Autodesk Inventor part; units mm, degrees
ref_plane "Work Plane1" through (104.775, 0, 0) normal (0, 0, -1) x (1, 0, 0)
ref_plane "YZ Plane" through (0, 0, 0) normal (1, 0, 0) x (0, 1, 0)
ref_plane "XZ Plane" through (0, 0, 0) normal (0, 1, 0) x (-1, 0, 0)
sketch "Sketch1" plane through (0, 0, 0) normal (0, 0, 1) x (1, 0, 0)
  line L0 (15.875, 0) -> (15.875, 2.413)
  line L1 (15.875, 2.413) -> (5.8717, 2.413)
  line L2 (5.8717, 2.413) -> (3.2258, 2.413)
  line L3 (0, 4.5593) -> (0, 1.8331)
  line L4 (0, 1.8331) -> (2.2098, 1.8331)
  line L5 (2.2098, 1.8331) -> (3.2681, 0)
  line L6 (3.2681, 0) -> (15.875, 0)
  line L7 (0, 4.5593) -> (0.7568, 4.5593)
  line L8 (0.7568, 4.5593) -> (3.2258, 2.413)
  line L9 (3.2258, 2.413) -> (3.2258, 2.413)
  line L10 (5.8717, 2.413) -> (3.2258, 2.413) construction
  line L11 (3.2258, 2.413) -> (3.2258, 2.413)
  line L12 (-3.175, 0) -> (19.05, 0)
  line L13 (0, -0.9119) -> (0, 5.4712)
  dimension "d0" = 15.875
  dimension "d1" = 10.0033
  dimension "d2" = 2.2098
  dimension "d3" = 4.826
  dimension "d6" = 3.2258
  dimension "d7" = 41
  dimension "d8" = 3.6662
  dimension "d9" = 60
  dimension "d10" = 9.1186
  dimension "d11" = 4.826
  dimension "d12" = 2.6459
revolve "Body" add sketch "Sketch1" angle 360 about axis through (3.2681, 0, 0) along (1, 0, 0) contours L6 L5 L4 L3 L7 L8 L2 L1 L0
sketch "Sketch2" plane through (0, 0, 0) normal (-1, 0, 0) x (0, 0, 1)
  circle A0 centre (0, 0) radius 1.8331
  line L0 (0, -6.383) -> (0, 6.383)
  line L1 (-6.383, 0) -> (6.383, 0)
  line L2 (1.8331, 0) -> (0.9165, -1.5875)
  line L3 (0.9165, -1.5875) -> (-0.9165, -1.5875)
  line L4 (-0.9165, -1.5875) -> (-1.8331, 0)
  line L5 (-1.8331, 0) -> (-0.9165, 1.5875)
  line L6 (-0.9165, 1.5875) -> (0.9165, 1.5875)
  line L7 (0.9165, 1.5875) -> (1.8331, 0)
  point P0 (0, 1.8331)
extrude "Slot" add sketch "Sketch2" against normal up to next contours L7 A0 | A0 L2 | L6 L0 A0 | A0 L0 L3 | L0 L6 A0 | A0 L3 L0 | L4 A0 | A0 L5
thread "Thread"
chamfer "Chamfer1" distance 0.6299 distance2 1.2598 1 edges at (15.875, -2.413, 0) measured on face at (15.875, -0.0132, -0.958)
ref_plane "Work Plane1" through (104.775, 0, 0) normal (0, 0, -1) x (1, 0, 0)
equation "\"d15\" = GEL"
equation "\"d17\" = -0.5 * SPD + 0.5 * GD"
equation "\"d18\" = GUL"
equation "\"d0\" = NLG"
equation "\"d1\" = GEL"
equation "\"d2\" = INTI"
equation "\"d3\" = GD"
equation "\"d6\" = KOH"
equation "\"d7\" = 0.5 * SEWI"
equation "\"d8\" = 1.1547 * SW"
equation "\"d10\" = KOD"
equation "\"d11\" = BDM"
equation "\"d12\" = GAL"
equation "\"NLG\" = 15.875"
equation "\"INTI\" = 2.2098"
equation "\"GEL\" = 10.00328"
equation "\"GAL\" = 2.64592"
equation "\"KOH\" = 3.2258"
equation "\"KOD\" = 9.1186"
equation "\"GUL\" = 1.25984"
equation "\"SPD\" = 3.56616"
equation "\"BDM\" = NND"
equation "\"GD\" = NND"
equation "\"SEWI\" = 82deg"
equation "\"SW\" = 3.175"
equation "\"TOA\" = 30deg"
equation "\"GD1\" = SPD"
equation "\"THREADDIA\" = 4.826"
equation "\"HHPTC\" = 1.05842"
equation "\"NND\" = 4.826"
equation "\"E0\" = 1.155 * SW"
properties part number "ANSI B18.3 - 10-24 UNC x 0.625" material "Steel, Mild"
Part model, mm, in its own coordinate system. A direction names the side the tool comes from. Coordinates: 2 decimals unless noted, no trailing zeros. Write each loop counter-clockwise with the first axis right and the second up, starting at its lowest first coordinate (ties: lowest second). Pieces come first, ordered by that corner, then holes.
Item 1: Which spindle directions (+Z, -Z, +X, -X, +Y, -Y) get a long thin tool onto all of the face, cutting with end or side? Do faces 4 (the face through (15.875, 0, 0)), 5 (the face through (1.159, 0.783, -1.381)). Say none if no direction does.
Item 2: Pin check, flat tips, straight feed: pin 1 (4 mm diameter, centred on x = 11.5, y = 3, fed in from -Z); pin 2 (4 mm diameter, centred on y = 1.5, z = 1, fed in from -X). Stop position of each tip, or through.
Item 3: Slice it at A-A (x = 5.25). Write the cut outline in (y, z), and give its area (3 significant figures).
Item 4: Mould opens along Y. For faces 1 (the face through (3.202, 0.053, 0.102)), 2 (the face through (0, 0, 2)), 3 (the face through (8.841, -1.915, 1.468)) say: released by +Y, released by -Y, zero draft, split by the parting line, or undercut.
Item 5: Probe line 1 (Z direction, x = 14.25, y = 0); line 2 (Y direction, x = 1.5, z = -0.5); line 3 (X direction, y = 1.25, z = 1) (3 decimals). List the from-to ranges inside material, lowest first.
Item 6: Slice it at B-B (x = 3). Write the cut outline in (y, z).
Results found:
1. face 4: +Z, -Z, +X, +Y, -Y
1. face 5: -X
2. pin 1: stops at z = -2.2
2. pin 2: stops at x = 0
3. outline: circle Ø4.83 at (0, 0)
3. area: 18.3 mm2
4. face 1: undercut
4. face 2: zero draft
4. face 3: split by the parting line
5. line 1: z = -2.41 to 2.41
5. line 2: y = -3.88 to -1.59, 1.59 to 3.88
5. line 3: x = 2.344 to 15.875
6. outline: circle Ø5.22 at (0, 0); hole circle Ø0.93 at (0, 0)
